The model under review builds one solid part; all positions refer to its coordinate system, in mm. Face numbers are marked on the shaded views. Give positions to 0.01 mm unless a question says otherwise; leave off trailing zeros. Order: outer loops, then holes, each group sorted by start corner. A loop starts at its lowest first (then second) coordinate and runs counter-clockwise, first axis right, second up. Notation, with made-up numbers: (52, 17) - (69, 17) arc R15 ccw to (69, 37) - close; hole circle Ø9 at (42.5, 50). An arc over 180 degrees is marked (long way). Put each result on its own line as item: value.
```python
from build123d import *

# Parameters (mm, degrees)
F1_ANGLE_BACK = 15
F1_ANGLE      = 30
F2_R          = 30


with BuildPart() as f1:
    # F0 (on Front) → F1 (revolve)
    with BuildSketch(Plane.XZ, mode=Mode.PRIVATE) as f1_sk:
        with BuildLine():
            Line((380, 0), (500, 0))
            ThreePointArc((500, 0), (494.9747468306, 70.7106781187), (480, 140))
            Line((480, 140), (364.8, 106.4))
            ThreePointArc((364.8, 106.4), (376.1808075912, 53.7401153702), (380, 0))
        make_face()
    revolve(f1_sk.sketch.rotate(Axis((0, 0, 25.3354795277), (0, 0, 1)), -F1_ANGLE_BACK), axis=Axis((0, 0, 25.3354795277), (0, 0, 1)), revolution_arc=F1_ANGLE)

    # F2
    f2_edges = [f1.edges().sort_by_distance(p)[0] for p in [
        (408.007069, -109.325165, 123.2),
        (425.007364, -113.88038, 0),
        (425.007364, 113.88038, 0),
        (408.007069, 109.325165, 123.2),
    ]]
    fillet(f2_edges, radius=F2_R)


solid = f1.part
```
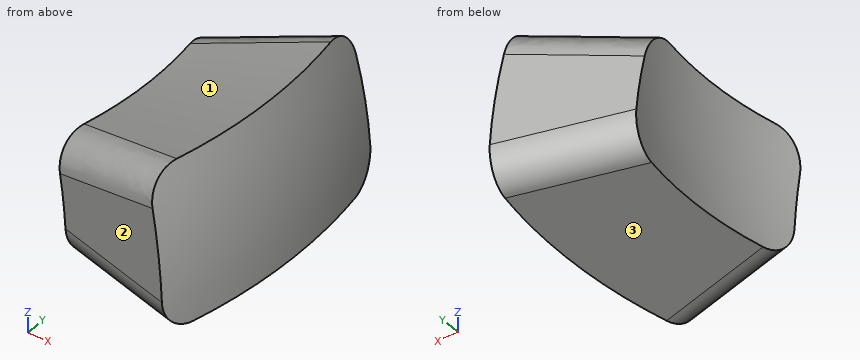
(1) Take a section at A-A, the plane z = 34. Write out the cut boundary in (x, y) (3 decimals).
The answers:
outline: (365.58, -97.957) - (481.845, -129.11) arc R498.843 ccw to (481.845, 129.11) - (365.58, 97.957) arc R378.476 cw to start
(2) The part is to be moulded in two halves that separate along Y. For the marked faces 1, 2 and 3, say which applies: pulls with the +Y half, pulls with the -Y half, needs draft (parallel to the pull), parting line crosses it, or undercut.
The answers:
face 1: undercut
face 2: pulls with the -Y half
face 3: needs draft
(3) Clearance check with flat-ended pins moving along their axes: pin 1 Ø2 at (y, z) = (83, 122.5) entering from +X; pin 2 Ø4 at (y, z) = (-36.5, 77) entering from +X; pin 3 Ø1 at (y, z) = (65, 123) entering from +X. State where each tip first meets the part, or that it passes through.
The answers:
pin 1: x = 477.91
pin 2: x = 493.03
pin 3: x = 480.4
(4) Wall thickness on L1, parallel to Y at x = 471, z = 55; L2, parallel to X at y = 19, z = 90.5; L3, parallel to Z at x = 465.5, y = 94: over which ranges is each line inside the solid? List them lowest first.
The answers:
L1: -126.2 to 126.2
L2: 368.58 to 491.37
L3: 0 to 138.51
